Design review of the part shown in the three views and the two pictorial views. Dimensions are in mm from the part's minimum x, y and z. Round coordinates to 2 decimals unless told otherwise and drop trailing zeros. Write each loop counter-clockwise with the first axis right and the second up, starting at its lowest first coordinate (ties: lowest second). Pieces come first, ordered by that corner, then holes. Notation, with made-up numbers: (44.25, 27) -> (81.25, 27) arc R30 cw to (81.25, 61) -> close; hole circle Ø5 at (-18, 41.5). An arc over 180 degrees is marked (long way). One line per question, with ' | ' between items. Start each with the question number.
1) Consider section C-C (y = 3). Give the boundary of the cut face in (x, z).
2) Consider section D-D (x = 10.5). Give the boundary of the cut face in (y, z) (1 decimal).
3) Consider section B-B (z = 0.5). Give the boundary of the cut face in (x, y).
4) For probe 1 along Y at (x, z) = (17, 0.95); probe 2 along Y at (x, z) = (10.5, 1.45) (1 decimal); probe 3 along Y at (x, z) = (15, 1.4), list the stretches that pass through material, from the lowest coordinate up.
5) Consider section A-A (x = 17). Give the boundary of the cut face in (y, z).
6) Mouldability with a two-part tool opening along Y and no side actions: class the marked faces 1, 2 and 3 as +Y half, -Y half, draft (parallel to the pull), parting line (faces both ways), or undercut.
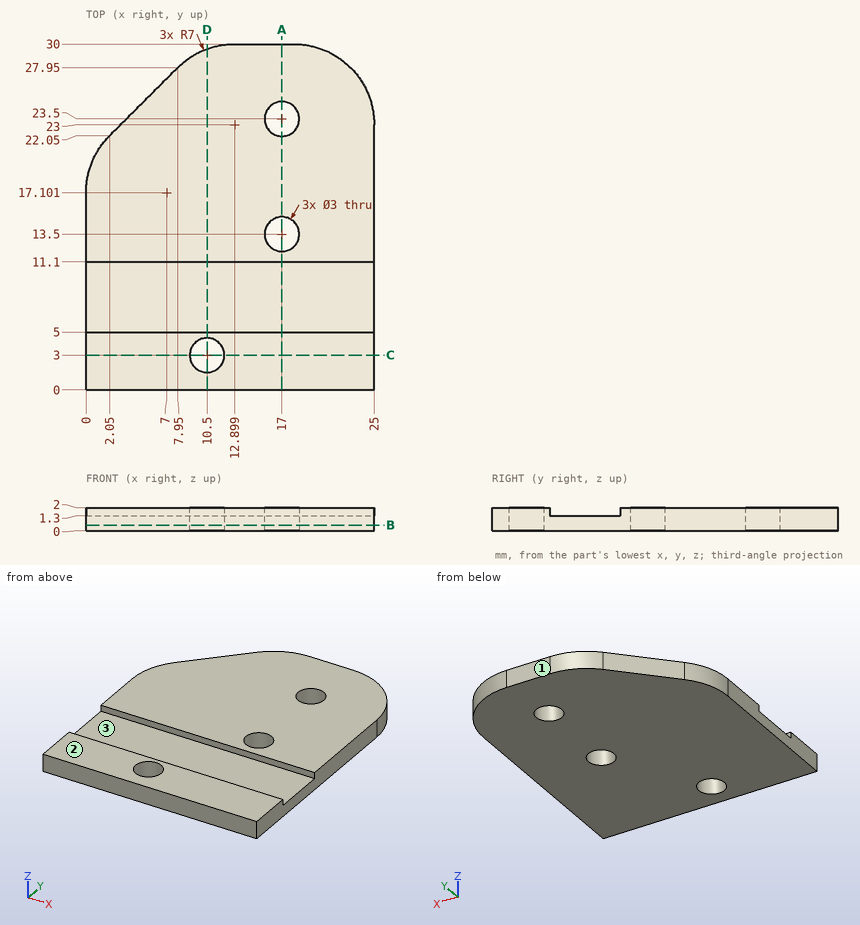
From the geometry:
1) outline: (0, 0) -> (9, 0) -> (9, 2) -> (0, 2) -> close; (12, 0) -> (25, 0) -> (25, 2) -> (12, 2) -> close
2) outline: (0, 0) -> (1.5, 0) -> (1.5, 2) -> (0, 2) -> close; (4.5, 0) -> (29.6, 0) -> (29.6, 2) -> (11.1, 2) -> (11.1, 1.3) -> (5, 1.3) -> (5, 2) -> (4.5, 2) -> close
3) outline: (0, 0) -> (25, 0) -> (25, 23) arc R7 ccw to (18, 30) -> (12.9, 30) arc R7 ccw to (7.95, 27.95) -> (2.05, 22.05) arc R7 ccw to (0, 17.1) -> close; hole circle Ø3 at (10.5, 3); hole circle Ø3 at (17, 13.5); hole circle Ø3 at (17, 23.5)
4) probe 1: y = 0 to 12, 15 to 22, 25 to 30 | probe 2: y = 0 to 1.5, 4.5 to 5, 11.1 to 29.6 | probe 3: y = 0 to 5, 11.1 to 30
5) outline: (0, 0) -> (12, 0) -> (12, 2) -> (11.1, 2) -> (11.1, 1.3) -> (5, 1.3) -> (5, 2) -> (0, 2) -> close; (15, 0) -> (22, 0) -> (22, 2) -> (15, 2) -> close; (25, 0) -> (30, 0) -> (30, 2) -> (25, 2) -> close
6) face 1: +Y half | face 2: draft | face 3: undercut
